from build123d import *

# Parameters (mm, degrees)
SKETCH1_W               = 12
SKETCH1_H               = 10
SKETCH1_R               = 1.5
SCREW_TABS_DEPTH        = 3
SCREW_TABS_2_DEPTH      = 3
SKETCH1_W_2             = 10
SKETCH1_H_2             = 12
SCREW_TABS_3_DEPTH      = 3
SKETCH2_W               = 3
SKETCH2_H               = 10
SKETCH2_H_2             = 11
SKETCH2_W_2             = 10
SKETCH2_H_3             = 3
VERTICAL_EXTRUDE_DEPTH  = 9
TOP_BRACKET_DEPTH       = 3
F_3MM_EDGE_ROUNDING_R   = 3
SKETCH4_R               = 3
SCREWHOLE_CLEARUP_DEPTH = 100.322706431


with BuildPart() as part:
    # Sketch1 → Screw tabs (new body)
    with BuildSketch(Plane(origin=(0, 0, 0), x_dir=(1, 0, 0), z_dir=(0, 1, 0))):
        with Locations((-69, 59)):
            Rectangle(SKETCH1_W, SKETCH1_H)
        with Locations(Location((-69, 59, 0), (0, 0, 270))):
            Circle(SKETCH1_R, mode=Mode.SUBTRACT)
    extrude(amount=SCREW_TABS_DEPTH)



with BuildPart() as body_2:
    # Sketch1 → Screw tabs 2 (new body)
    with BuildSketch(Plane(origin=(0, 0, 0), x_dir=(1, 0, 0), z_dir=(0, 1, 0))):
        with Locations((27, 59)):
            Rectangle(SKETCH1_W, SKETCH1_H)
        with Locations(Location((27, 59, 0), (0, 0, 270))):
            Circle(SKETCH1_R, mode=Mode.SUBTRACT)
    extrude(amount=SCREW_TABS_2_DEPTH)


with BuildPart() as body_3:
    # Sketch1 → Screw tabs 3 (new body)
    with BuildSketch(Plane(origin=(0, 0, 0), x_dir=(1, 0, 0), z_dir=(0, 1, 0))):
        Rectangle(SKETCH1_W_2, SKETCH1_H_2)
        with Locations(Location((0, 0, 0), (0, 0, 270))):
            Circle(SKETCH1_R, mode=Mode.SUBTRACT)
    extrude(amount=SCREW_TABS_3_DEPTH)


with BuildPart() as part_1:
    add(part.part)

    add(body_2.part)  # Vertical extrude merges body 2

    add(body_3.part)  # Vertical extrude merges body 3
    # Sketch2 → Vertical extrude (add)
    with BuildSketch(Plane(origin=(0, 3, 0), x_dir=(1, 0, 0), z_dir=(0, 1, 0))):
        with Locations((-64.5, 59)):
            Rectangle(SKETCH2_W, SKETCH2_H)
        with Locations((22.5, 58.5)):
            Rectangle(SKETCH2_W, SKETCH2_H_2)
        with Locations((0, 4.5)):
            Rectangle(SKETCH2_W_2, SKETCH2_H_3)
    extrude(amount=VERTICAL_EXTRUDE_DEPTH)

    # Sketch3 → Top bracket (add)
    with BuildSketch(Plane(origin=(0, 12, 0), x_dir=(1, 0, 0), z_dir=(0, 1, 0))):
        with BuildLine():
            Line((-66, 64), (24, 64))
            Line((24, 64), (24, 53))
            Line((24, 53), (10, 53))
            ThreePointArc((10, 53), (6.464466094, 51.535533906), (5, 48))
            Line((5, 48), (5, 3))
            Line((5, 3), (-5, 3))
            Line((-5, 3), (-5, 48))
            ThreePointArc((-5, 48), (-6.464466094, 51.535533906), (-10, 53))
            Line((-10, 53), (-66, 53))
            Line((-66, 53), (-66, 64))
        make_face()
    extrude(amount=TOP_BRACKET_DEPTH)

    # 3mm edge rounding
    # the kernel refuses this fillet: 3 mm, written as the material it adds along each edge
    with BuildSketch(Plane(origin=(24, 3, -64), x_dir=(1, 0, 0), z_dir=(0, 0, 1))) as f_3mm_edge_rounding_piece_1_section:
        with BuildLine():
            CenterArc((F_3MM_EDGE_ROUNDING_R, F_3MM_EDGE_ROUNDING_R), F_3MM_EDGE_ROUNDING_R, 180, 90)
            Line((0, F_3MM_EDGE_ROUNDING_R), (0, 0))
            Line((0, 0), (F_3MM_EDGE_ROUNDING_R, 0))
        make_face()
    f_3mm_edge_rounding_piece_1 = extrude(amount=10, mode=Mode.PRIVATE)
    f_3mm_edge_rounding_piece_1 = f_3mm_edge_rounding_piece_1 - Plane(origin=(27, 3.680423694, -59), x_dir=(0, 0, 1), z_dir=(0, -1, 0)) * Cylinder(1.5, 33, mode=Mode.PRIVATE)
    add(f_3mm_edge_rounding_piece_1)
    with BuildSketch(Plane(origin=(5, 3, -3), x_dir=(0, 0, 1), z_dir=(-1, 0, 0))) as f_3mm_edge_rounding_piece_2_section:
        with BuildLine():
            CenterArc((F_3MM_EDGE_ROUNDING_R, F_3MM_EDGE_ROUNDING_R), F_3MM_EDGE_ROUNDING_R, 180, 90)
            Line((0, F_3MM_EDGE_ROUNDING_R), (0, 0))
            Line((0, 0), (F_3MM_EDGE_ROUNDING_R, 0))
        make_face()
    f_3mm_edge_rounding_piece_2 = extrude(amount=10, mode=Mode.PRIVATE)
    f_3mm_edge_rounding_piece_2 = f_3mm_edge_rounding_piece_2 - Plane(origin=(0, 3.680423694, 0), x_dir=(0, 0, 1), z_dir=(0, -1, 0)) * Cylinder(1.5, 32, mode=Mode.PRIVATE)
    add(f_3mm_edge_rounding_piece_2)
    with BuildSketch(Plane(origin=(-66, 3, -64), x_dir=(0, 1, 0), z_dir=(0, 0, 1))) as f_3mm_edge_rounding_piece_3_section:
        with BuildLine():
            CenterArc((F_3MM_EDGE_ROUNDING_R, F_3MM_EDGE_ROUNDING_R), F_3MM_EDGE_ROUNDING_R, 180, 90)
            Line((0, F_3MM_EDGE_ROUNDING_R), (0, 0))
            Line((0, 0), (F_3MM_EDGE_ROUNDING_R, 0))
        make_face()
    f_3mm_edge_rounding_piece_3 = extrude(amount=10, mode=Mode.PRIVATE)
    f_3mm_edge_rounding_piece_3 = f_3mm_edge_rounding_piece_3 - Plane(origin=(-69, 3.680423205, -59), x_dir=(0, 0, 1), z_dir=(0, -1, 0)) * Cylinder(1.5, 32, mode=Mode.PRIVATE)
    add(f_3mm_edge_rounding_piece_3)
    # the kernel refuses this fillet: 3 mm, written as the material it takes off along each edge
    with BuildSketch(Plane(origin=(-63, 0, -71.5), x_dir=(0, 1, 0), z_dir=(0, 0, 1)), Plane(origin=(21, 0, -46.5), x_dir=(0, 1, 0), z_dir=(0, 0, -1))) as f_3mm_edge_rounding_2_piece_1:
        with BuildLine():
            CenterArc((F_3MM_EDGE_ROUNDING_R, F_3MM_EDGE_ROUNDING_R), F_3MM_EDGE_ROUNDING_R, 180, 90)
            Line((0, F_3MM_EDGE_ROUNDING_R), (0, 0))
            Line((0, 0), (F_3MM_EDGE_ROUNDING_R, 0))
        make_face()
    extrude(amount=25, mode=Mode.SUBTRACT)
    with BuildSketch(Plane(origin=(33, -7.5, -64), x_dir=(-1, 0, 0), z_dir=(0, 1, 0)), Plane(origin=(5, -7.5, 6), x_dir=(0, 0, -1), z_dir=(0, 1, 0)), Plane(origin=(-75, -7.5, -54), x_dir=(1, 0, 0), z_dir=(0, 1, 0))) as f_3mm_edge_rounding_2_piece_2:
        with BuildLine():
            CenterArc((F_3MM_EDGE_ROUNDING_R, F_3MM_EDGE_ROUNDING_R), F_3MM_EDGE_ROUNDING_R, 180, 90)
            Line((0, F_3MM_EDGE_ROUNDING_R), (0, 0))
            Line((0, 0), (F_3MM_EDGE_ROUNDING_R, 0))
        make_face()
    extrude(amount=18, mode=Mode.SUBTRACT)
    with BuildSketch(Plane(origin=(33, -7.5, -54), x_dir=(-1, 0, 0), z_dir=(0, 1, 0)), Plane(origin=(-5, -7.5, 6), x_dir=(0, 0, -1), z_dir=(0, 1, 0)), Plane(origin=(-75, -7.5, -64), x_dir=(1, 0, 0), z_dir=(0, 1, 0))) as f_3mm_edge_rounding_2_piece_3:
        with BuildLine():
            CenterArc((F_3MM_EDGE_ROUNDING_R, -F_3MM_EDGE_ROUNDING_R), F_3MM_EDGE_ROUNDING_R, 90, 90)
            Line((0, -F_3MM_EDGE_ROUNDING_R), (0, 0))
            Line((0, 0), (F_3MM_EDGE_ROUNDING_R, 0))
        make_face()
    extrude(amount=18, mode=Mode.SUBTRACT)
    with BuildSketch(Plane(origin=(24, 15, -71.5), x_dir=(-1, 0, 0), z_dir=(0, 0, 1)), Plane(origin=(-66, 15, -45.5), x_dir=(1, 0, 0), z_dir=(0, 0, -1))) as f_3mm_edge_rounding_2_piece_4:
        with BuildLine():
            CenterArc((F_3MM_EDGE_ROUNDING_R, F_3MM_EDGE_ROUNDING_R), F_3MM_EDGE_ROUNDING_R, 180, 90)
            Line((0, F_3MM_EDGE_ROUNDING_R), (0, 0))
            Line((0, 0), (F_3MM_EDGE_ROUNDING_R, 0))
        make_face()
    extrude(amount=26, mode=Mode.SUBTRACT)
    with BuildSketch(Plane(origin=(12.5, 15, -3), x_dir=(0, -1, 0), z_dir=(-1, 0, 0))) as f_3mm_edge_rounding_2_piece_5:
        with BuildLine():
            CenterArc((F_3MM_EDGE_ROUNDING_R, -F_3MM_EDGE_ROUNDING_R), F_3MM_EDGE_ROUNDING_R, 90, 90)
            Line((0, -F_3MM_EDGE_ROUNDING_R), (0, 0))
            Line((0, 0), (F_3MM_EDGE_ROUNDING_R, 0))
        make_face()
    extrude(amount=25, mode=Mode.SUBTRACT)

    # Sketch4 → Screwhole clearup (cut, through all)
    with BuildSketch(Plane(origin=(0, 3, 0), x_dir=(1, 0, 0), z_dir=(0, 1, 0))):
        with Locations((-69, 59)):
            Circle(SKETCH4_R)
        Circle(SKETCH4_R)
        with Locations((27, 59)):
            Circle(SKETCH4_R)
    extrude(amount=SCREWHOLE_CLEARUP_DEPTH, mode=Mode.SUBTRACT)


solid = part_1.part
Here's how the part is built. I have some questions about the finished solid (model axes, mm). A direction names the side the tool comes from. Coordinates: 2 decimals unless noted, no trailing zeros. Loops run counter-clockwise (first coordinate to the right, second up) from the corner with the lowest first, then second, coordinate; pieces in that order, holes last.
1. If we mould it in two halves opening along X, with no side actions, what happens to faces 1 (the flat face through (0, 3, 2)), 2 (the flat face through (29, 3, -59)), 3 (the cylindrical face through (-66.562, 4.252, -62.091))? For each: pulls with the +X half, pulls with the -X half, needs draft (parallel to the pull), parting line crosses it, or undercut.
2. Imagine slicing it at A-A, the plane z = -25.5. Please give me the cut outline in (x, y).
3. Imagine slicing it at B-B, the plane x = -39. Please give me the cut outline in (y, z), and give its area (3 significant figures).
4. For P1, Ø7, axis at x = 27, z = -57.5, coming from the +Y side; P2, Ø3, axis at x = 1, z = -16, coming from the -Y side; P3, Ø6, axis at x = -17.5, y = 7.5, coming from the -Z side; P4, Ø10, axis at x = -1, z = -0.5, coming from the +Y side, each with a flat end and sliding along its axis, tell me the tip position at first contact or that it passes through.
5. I need wall thicknesses on L1, parallel to Z at x = 27, y = 0.75; L2, parallel to Z at x = 0, y = 1.05; L3, parallel to X at y = 1.35, z = 0. Which ranges of each line are inside material? Lowest first, please.
6. For faces 4 (the flat face through (-72, 3, -59)), 5 (the cylindrical face through (21.9, 0.86, -58.93)), 6 (the cylindrical face through (24, 4, -59)), which set-ups out of +Z, -Z, +X, -X, +Y, -Y let a thin tool reach every point of the face, with its end or its side?
Taken from the geometry:
1. face 1: undercut
1. face 2: needs draft
1. face 3: pulls with the -X half
2. outline: (-5, 12) - (5, 12) - (5, 15) - (-5, 15) - close
3. outline: (12, -64) - (15, -64) - (15, -53) - (12, -53) - close
3. area: 33.0 mm2
4. P1: stops at y = 13.66
4. P2: stops at y = 12
4. P3: passes through
4. P4: stops at y = 14.96
5. L1: z = -64 to -60.5, -57.5 to -54
5. L2: z = -6 to -1.5, 1.5 to 6
5. L3: x = -5 to -1.5, 1.5 to 5
6. face 4: -X, +Y
6. face 5: +Z, -Z, -Y
6. face 6: +X, +Y
